```python
from build123d import *

# Parameters (mm, degrees)
F0_R      = 7.5
F1_DEPTH  = 25
F2_R      = 5.5
F3_DEPTH  = 20
F4_R      = 1.5
F5_DEPTH  = 5
F6_R      = 1.5
F7_DEPTH  = 7.501
F8_R      = 0.9
F9_DEPTH  = 7.501
F10_R     = 1.5
F11_DEPTH = 7.501
F12_R     = 0.9
F13_DEPTH = 7.501


with BuildPart() as f1:
    # F0 (on Front) → F1 (new body)
    with BuildSketch(Plane.XZ):
        Circle(F0_R)
    extrude(amount=F1_DEPTH)

    # F2 (on face) → F3 (cut)
    with BuildSketch(Plane.XZ.offset(25)):
        Circle(F2_R)
    extrude(amount=-F3_DEPTH, mode=Mode.SUBTRACT)

    # F4 (on face) → F5 (cut, through all)
    with BuildSketch(Plane.XZ.offset(5)):
        Circle(F4_R)
    extrude(amount=-F5_DEPTH, mode=Mode.SUBTRACT)

    # F6 (on Top) → F7 (cut, through all)
    with BuildSketch(Plane.XY):
        with Locations((0, -20.5)):
            Circle(F6_R)
    extrude(amount=F7_DEPTH, mode=Mode.SUBTRACT)

    # F8 (on Top) → F9 (cut, through all)
    with BuildSketch(Plane.XY):
        with Locations((0, -20.5)):
            Circle(F8_R)
    extrude(amount=-F9_DEPTH, mode=Mode.SUBTRACT)

    # F10 (on Right) → F11 (cut, through all)
    with BuildSketch(Plane.YZ):
        with Locations((-20.5, 0)):
            Circle(F10_R)
    extrude(amount=-F11_DEPTH, mode=Mode.SUBTRACT)

    # F12 (on Right) → F13 (cut, through all)
    with BuildSketch(Plane.YZ):
        with Locations((-20.5, 0)):
            Circle(F12_R)
    extrude(amount=F13_DEPTH, mode=Mode.SUBTRACT)


solid = f1.part
```
The listing builds one solid part. Answer for the finished solid, in the listing's coordinates (mm). A direction names the side the tool comes from. Give positions to 0.01 mm unless a question says otherwise; leave off trailing zeros. Order: outer loops, then holes, each group sorted by start corner. A loop starts at its lowest first (then second) coordinate and runs counter-clockwise, first axis right, second up. Notation, with made-up numbers: (25, -28.75) - (52, -28.75) arc R10 ccw to (52, -20.75) - close; hole circle Ø6 at (61, 15.5). An arc over 180 degrees is marked (long way). Use one line per item in the form item = value. Start each with the question number.
(1) Flat-ended cylindrical pins translate along their axes: pin 1 Ø2.5 at (x, z) = (0, 0) entering from -Y; pin 2 Ø2.5 at (x, y) = (0, -20.5) entering from +Z; pin 3 Ø1.5 at (x, y) = (4.5, -21) entering from -Z; pin 4 Ø1.5 at (y, z) = (-7, -2) entering from +X. Find the tip coordinate at first contact, or state that the pin passes through.
(2) A cutting plane is placed at A-A, the plane z = 0. Write down the section's boundary in (x, y).
(3) A cutting plane is placed at D-D, the plane z = -2. Write down the section's boundary in (x, y).
(4) A cutting plane is placed at C-C, the plane y = -20.5. Write down the section's boundary in (x, z).
(5) For faces 4 (the cylindrical face through (-1.2, -21.4, 6.4)), 5 (the flat face through (-1.3, -5, -1.1)), 6 (the flat face through (2, 0, 0)), determine the directions among +Z, -Z, +X, -X, +Y, -Y from which every point of the face is accessible in a straight line to the end or side of a thin tool.
(6) Consider line 1 (Z direction, x = 0, y = -17.5); line 2 (Y direction, x = 0, z = -6.5); line 3 (Z direction, x = 0, y = -3.7). Determine where each line is inside the solid, lowest interval first. Write a range as from..to.
(7) A cutting plane is placed at B-B, the plane x = 0. Write down the section's boundary in (y, z), then the cut area to 3 significant figures.
(8) The mould has two halves that part along X. Classify faces 1 (the cylindrical face through (-6, -19, 0)), 2 (the cylindrical face through (2.5, -15.1, -4.9)), 3 (the cylindrical face through (6.93, -12.32, -2.87)): released by +X, released by -X, zero draft, split by the parting line, or undercut.
Ans:
q1.pin_1 = through
q1.pin_2 = -5.36
q1.pin_3 = -6.5
q1.pin_4 = 7.4
q2.outline = (-7.5, -25) - (-5.5, -25) - (-5.5, -22) - (-7.5, -22) - close; (-7.5, -19) - (-5.5, -19) - (-5.5, -5) - (-1.5, -5) - (-1.5, 0) - (-7.5, 0) - close; (1.5, -5) - (5.5, -5) - (5.5, -19.6) - (7.5, -19.6) - (7.5, 0) - (1.5, 0) - close; (5.5, -25) - (7.5, -25) - (7.5, -21.4) - (5.5, -21.4) - close
q3.outline = (-7.23, -25) - (-5.12, -25) - (-5.12, -5) - (5.12, -5) - (5.12, -25) - (7.23, -25) - (7.23, 0) - (-7.23, 0) - close
q4.outline = (-7.35, -1.5) arc R7.5 ccw to (-0.9, -7.45) - (-0.9, -5.43) arc R5.5 cw to (-5.29, -1.5) - close; (-7.35, 1.5) - (-5.29, 1.5) arc R5.5 cw to (-1.5, 5.29) - (-1.5, 7.35) arc R7.5 ccw to start; (0.9, -7.45) arc R7.5 ccw to (7.45, -0.9) - (5.43, -0.9) arc R5.5 cw to (0.9, -5.43) - close; (1.5, 5.29) arc R5.5 cw to (5.43, 0.9) - (7.45, 0.9) arc R7.5 ccw to (1.5, 7.35) - close
q5.face_4 = +Z
q5.face_5 = -Y
q5.face_6 = +Z, -Z, +X, -X, +Y
q6.line_1 = -7.5..-5.5, 5.5..7.5
q6.line_2 = -25..-21.4, -19.6..0
q6.line_3 = -7.5..-1.5, 1.5..7.5
q7.outline = (-25, -7.5) - (-21.4, -7.5) - (-21.4, -5.5) - (-25, -5.5) - close; (-25, 5.5) - (-22, 5.5) - (-22, 7.5) - (-25, 7.5) - close; (-19.6, -7.5) - (0, -7.5) - (0, -1.5) - (-5, -1.5) - (-5, -5.5) - (-19.6, -5.5) - close; (-19, 5.5) - (-5, 5.5) - (-5, 1.5) - (0, 1.5) - (0, 7.5) - (-19, 7.5) - close
q7.area = 130 mm^2
q8.face_1 = zero draft
q8.face_2 = undercut
q8.face_3 = split by the parting line
